Can you work these out from the model? Positions are in its coordinate system, mm. Face numbers are marked on the shaded views. A direction names the side the tool comes from. Round coordinates to 2 decimals unless told otherwise and drop trailing zeros. Order: outer loops, then holes, each group sorted by start corner. A loop starts at its lowest first (then second) coordinate and runs counter-clockwise, first axis right, second up. Notation, with made-up numbers: M 75.25,-31 L 111.25,-31 A17 cw 111.25,-16 Z; hole C 82.25,25.5 d11. An arc over 180 degrees is marked long. One line per question, with ' | ' between items.
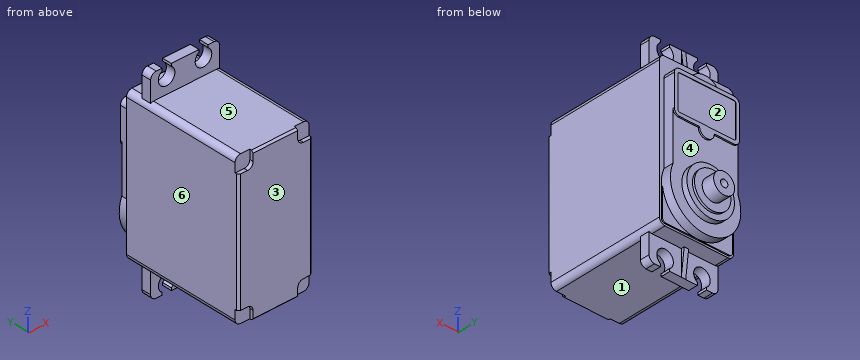
```python
from build123d import *

# Parameters (mm, degrees)
BOSS_EXTRUDE1_DEPTH  = 33.2
BOSS_EXTRUDE2_DEPTH  = 2.55
BOSS_EXTRUDE11_DEPTH = 0.3
BOSS_EXTRUDE3_DEPTH  = 2.7
SKETCH6_R            = 4.4225
BOSS_EXTRUDE4_DEPTH  = 2.5
SKETCH7_R            = 6.45
BOSS_EXTRUDE5_DEPTH  = 1.5
SKETCH8_R            = 4.95
BOSS_EXTRUDE6_DEPTH  = 0.6
SKETCH10_R           = 2.85
BOSS_EXTRUDE7_DEPTH  = 3.4
SKETCH12_R           = 1
CUT_EXTRUDE1_DEPTH   = 5
BOSS_EXTRUDE9_DEPTH  = 0.4
BOSS_EXTRUDE10_DEPTH = 0.3
CHAMFER1_SIZE        = 0.5
CUT_EXTRUDE2_DEPTH   = 1
MIRROR2_COPY_1_DEPTH = 1
BOSS_EXTRUDE12_DEPTH = 0.6


with BuildPart() as part:
    # Sketch1 → Boss-Extrude1 (new body)
    with BuildSketch(Plane(origin=(0, 0, 0), x_dir=(1, 0, 0), z_dir=(0, 1, 0))):
        with BuildLine():
            Line((-8.55, -25.58), (8.55, -25.58))
            ThreePointArc((8.55, -25.58), (9.610660172, -25.140660172), (10.05, -24.08))
            Line((10.05, -24.08), (10.05, 13.72))
            ThreePointArc((10.05, 13.72), (9.610660172, 14.780660172), (8.55, 15.22))
            Line((8.55, 15.22), (-8.55, 15.22))
            ThreePointArc((-8.55, 15.22), (-9.610660172, 14.780660172), (-10.05, 13.72))
            Line((-10.05, 13.72), (-10.05, -24.08))
            ThreePointArc((-10.05, -24.08), (-9.610660172, -25.140660172), (-8.55, -25.58))
        make_face()
    extrude(amount=BOSS_EXTRUDE1_DEPTH)

    # Sketch4 → Boss-Extrude2 (add)
    with BuildSketch(Plane(origin=(0, 26.8, 0), x_dir=(1, 0, 0), z_dir=(0, 1, 0))):
        with BuildLine():
            Line((-6.25, 22.12), (-6.25, 21.440828693))
            ThreePointArc((-6.25, 21.440828693), (-5, 17.32), (-3.75, 21.440828693))
            Line((-3.75, 21.440828693), (-3.75, 22.12))
            Line((-3.75, 22.12), (3.75, 22.12))
            Line((3.75, 22.12), (3.75, 21.440828693))
            ThreePointArc((3.75, 21.440828693), (5, 17.32), (6.25, 21.440828693))
            Line((6.25, 21.440828693), (6.25, 22.12))
            Line((6.25, 22.12), (7.85, 22.12))
            ThreePointArc((7.85, 22.12), (8.910660172, 21.680660172), (9.35, 20.62))
            Line((9.35, 20.62), (9.35, -30.98))
            ThreePointArc((9.35, -30.98), (8.910660172, -32.040660172), (7.85, -32.48))
            Line((7.85, -32.48), (6.25, -32.48))
            Line((6.25, -32.48), (6.25, -31.800828693))
            ThreePointArc((6.25, -31.800828693), (5, -27.68), (3.75, -31.800828693))
            Line((3.75, -31.800828693), (3.75, -32.48))
            Line((3.75, -32.48), (-3.75, -32.48))
            Line((-3.75, -32.48), (-3.75, -31.800828693))
            ThreePointArc((-3.75, -31.800828693), (-5, -27.68), (-6.25, -31.800828693))
            Line((-6.25, -31.800828693), (-6.25, -32.48))
            Line((-6.25, -32.48), (-7.85, -32.48))
            ThreePointArc((-7.85, -32.48), (-8.910660172, -32.040660172), (-9.35, -30.98))
            Line((-9.35, -30.98), (-9.35, 20.62))
            ThreePointArc((-9.35, 20.62), (-8.910660172, 21.680660172), (-7.85, 22.12))
            Line((-7.85, 22.12), (-6.25, 22.12))
        make_face()
    extrude(amount=BOSS_EXTRUDE2_DEPTH)

    # Sketch16 → Boss-Extrude11 (add)
    with BuildSketch(Plane(origin=(0, 33.2, 0), x_dir=(1, 0, 0), z_dir=(0, 1, 0))):
        with BuildLine():
            Line((-9.55, 13.72), (-9.55, 6.17))
            Line((-9.55, 6.17), (9.55, 6.17))
            Line((9.55, 6.17), (9.55, 13.72))
            ThreePointArc((9.55, 13.72), (9.257106781, 14.427106781), (8.55, 14.72))
            Line((8.55, 14.72), (-8.55, 14.72))
            ThreePointArc((-8.55, 14.72), (-9.257106781, 14.427106781), (-9.55, 13.72))
        make_face()
    extrude(amount=BOSS_EXTRUDE11_DEPTH)

    # Sketch5 → Boss-Extrude3 (add)
    with BuildSketch(Plane(origin=(0, 33.2, 0), x_dir=(1, 0, 0), z_dir=(0, 1, 0))):
        with BuildLine():
            Line((-8.85, 1.581128311), (-8.85, -20.08))
            ThreePointArc((-8.85, -20.08), (-8.410660172, -21.140660172), (-7.35, -21.58))
            Line((-7.35, -21.58), (7.35, -21.58))
            ThreePointArc((7.35, -21.58), (8.410660172, -21.140660172), (8.85, -20.08))
            Line((8.85, -20.08), (8.85, 1.581128311))
            ThreePointArc((8.85, 1.581128311), (0, 14.72), (-8.85, 1.581128311))
        make_face()
    extrude(amount=BOSS_EXTRUDE3_DEPTH)

    # Sketch6 → Boss-Extrude4 (add)
    with BuildSketch(Plane(origin=(0, 33.2, 0), x_dir=(1, 0, 0), z_dir=(0, 1, 0))):
        with Locations((0, -19.1575)):
            Circle(SKETCH6_R)
    extrude(amount=BOSS_EXTRUDE4_DEPTH)

    # Sketch7 → Boss-Extrude5 (add)
    with BuildSketch(Plane(origin=(0, 35.9, 0), x_dir=(1, 0, 0), z_dir=(0, 1, 0))):
        with Locations((0, 5.17)):
            Circle(SKETCH7_R)
    extrude(amount=BOSS_EXTRUDE5_DEPTH)

    # Sketch8 → Boss-Extrude6 (add)
    with BuildSketch(Plane(origin=(0, 37.4, 0), x_dir=(1, 0, 0), z_dir=(0, 1, 0))):
        with Locations((0, 5.17)):
            Circle(SKETCH8_R)
    extrude(amount=BOSS_EXTRUDE6_DEPTH)

    # Sketch10 → Boss-Extrude7 (add)
    with BuildSketch(Plane(origin=(0, 38, 0), x_dir=(1, 0, 0), z_dir=(0, 1, 0))):
        with Locations((0, 5.17)):
            Circle(SKETCH10_R)
    extrude(amount=BOSS_EXTRUDE7_DEPTH)

    # Sketch12 → Cut-Extrude1 (cut)
    with BuildSketch(Plane(origin=(0, 41.4, 0), x_dir=(1, 0, 0), z_dir=(0, 1, 0))):
        with Locations((0, 5.17)):
            Circle(SKETCH12_R)
    extrude(amount=-CUT_EXTRUDE1_DEPTH, mode=Mode.SUBTRACT)

    # Sketch13 → Boss-Extrude9 (add)
    with BuildSketch(Plane(origin=(0, 35.9, 0), x_dir=(1, 0, 0), z_dir=(0, 1, 0))):
        with BuildLine():
            Line((-8.85, -11.58), (-8.85, -20.08))
            ThreePointArc((-8.85, -20.08), (-8.410660172, -21.140660172), (-7.35, -21.58))
            Line((-7.35, -21.58), (7.35, -21.58))
            ThreePointArc((7.35, -21.58), (8.410660172, -21.140660172), (8.85, -20.08))
            Line((8.85, -20.08), (8.85, -11.58))
            ThreePointArc((8.85, -11.58), (8.410660172, -10.519339828), (7.35, -10.08))
            Line((7.35, -10.08), (2, -10.08))
            ThreePointArc((2, -10.08), (0, -8.08), (-2, -10.08))
            Line((-2, -10.08), (-7.35, -10.08))
            ThreePointArc((-7.35, -10.08), (-8.410660172, -10.519339828), (-8.85, -11.58))
        make_face()
        with BuildLine():
            Line((-7.85, -11.58), (-7.85, -20.08))
            ThreePointArc((-7.85, -20.08), (-7.703553391, -20.433553391), (-7.35, -20.58))
            Line((-7.35, -20.58), (7.35, -20.58))
            ThreePointArc((7.35, -20.58), (7.703553391, -20.433553391), (7.85, -20.08))
            Line((7.85, -20.08), (7.85, -11.58))
            ThreePointArc((7.85, -11.58), (7.703553391, -11.226446609), (7.35, -11.08))
            Line((7.35, -11.08), (-7.35, -11.08))
            ThreePointArc((-7.35, -11.08), (-7.703553391, -11.226446609), (-7.85, -11.58))
        make_face(mode=Mode.SUBTRACT)
    extrude(amount=BOSS_EXTRUDE9_DEPTH)

    # Sketch14 → Boss-Extrude10 (add)
    with BuildSketch(Plane(origin=(0, 35.9, 0), x_dir=(1, 0, 0), z_dir=(0, 1, 0))):
        with BuildLine():
            Line((-7.85, -11.58), (-7.85, -20.08))
            ThreePointArc((-7.85, -20.08), (-7.703553391, -20.433553391), (-7.35, -20.58))
            Line((-7.35, -20.58), (7.35, -20.58))
            ThreePointArc((7.35, -20.58), (7.703553391, -20.433553391), (7.85, -20.08))
            Line((7.85, -20.08), (7.85, -11.58))
            ThreePointArc((7.85, -11.58), (7.703553391, -11.226446609), (7.35, -11.08))
            Line((7.35, -11.08), (-7.35, -11.08))
            ThreePointArc((-7.35, -11.08), (-7.703553391, -11.226446609), (-7.85, -11.58))
        make_face()
    extrude(amount=BOSS_EXTRUDE10_DEPTH)

    # Chamfer1
    chamfer1_edges = [part.edges().sort_by_distance(p)[0] for p in [
        (-10.05, 0, 5.18),
        (-9.610660172, 0, -14.780660172),
        (0, 0, -15.22),
        (9.610660172, 0, -14.780660172),
        (10.05, 0, 5.18),
        (9.610660172, 0, 25.140660172),
        (0, 0, 25.58),
        (-9.610660172, 0, 25.140660172),
    ]]
    chamfer(chamfer1_edges, length=CHAMFER1_SIZE)

    # Sketch17 → Cut-Extrude2 (cut)
    with BuildSketch(Plane.XZ):
        with BuildLine():
            Line((-10.05, 21.58), (-10.05, 24.08))
            ThreePointArc((-10.05, 24.08), (-9.610660172, 25.140660172), (-8.55, 25.58))
            Line((-8.55, 25.58), (-6.05, 25.58))
            Line((-6.05, 25.58), (-6.05, 23.08))
            ThreePointArc((-6.05, 23.08), (-6.489339828, 22.019339828), (-7.55, 21.58))
            Line((-7.55, 21.58), (-10.05, 21.58))
        make_face()
    cut_extrude2 = extrude(amount=-CUT_EXTRUDE2_DEPTH, mode=Mode.SUBTRACT)

    # Mirror1: Cut-Extrude2 across plane
    add(cut_extrude2.mirror(Plane(origin=(0, 0, 0), x_dir=(0, 0, 1), z_dir=(1, 0, 0))), mode=Mode.SUBTRACT)

    # Mirror2: Cut-Extrude2 across plane
    add(cut_extrude2.mirror(Plane.XY.offset(5.18)), mode=Mode.SUBTRACT)

    # Mirror2 copy 1 sketch → Mirror2 copy 1 (cut)
    with BuildSketch(Plane(origin=(0, 0, 10.36), x_dir=(-1, 0, 0), z_dir=(0, -1, 0))):
        with BuildLine():
            Line((-10.05, 21.58), (-10.05, 24.08))
            ThreePointArc((-10.05, 24.08), (-9.610660172, 25.140660172), (-8.55, 25.58))
            Line((-8.55, 25.58), (-6.05, 25.58))
            Line((-6.05, 25.58), (-6.05, 23.08))
            ThreePointArc((-6.05, 23.08), (-6.489339828, 22.019339828), (-7.55, 21.58))
            Line((-7.55, 21.58), (-10.05, 21.58))
        make_face()
    extrude(amount=-MIRROR2_COPY_1_DEPTH, mode=Mode.SUBTRACT)

    # Sketch19 → Boss-Extrude12 (add, symmetric)
    with BuildSketch(Plane(origin=(0, 0, 0), x_dir=(0, 0, -1), z_dir=(1, 0, 0))):
        Polygon((-25.58, 30.2), (-25.58, 29.35), (-32.48, 29.35), align=None)
        Polygon((15.22, 30.2), (15.22, 29.35), (22.12, 29.35), align=None)
    extrude(amount=BOSS_EXTRUDE12_DEPTH, both=True)


solid = part.part
```
(1) Will these pins go through, and if not, where does the flat tip stop? pin 1 Ø0.6 at (x, z) = (0, -5) entering from +Y; pin 2 Ø6 at (x, y) = (7, 11) entering from -Z; pin 3 Ø5 at (x, y) = (4.5, 33.5) entering from +Z.
Final values:
pin 1: y = 36.4 | pin 2: z = -15.22 | pin 3: z = 25.58
(2) If we section it at C-C on z = -19.57: Please give me the cut outline in (x, y).
Final values:
outline: M -9.35,26.8 L -7.25,26.8 L -7.25,29.35 L -9.35,29.35 Z; M -2.75,26.8 L 2.75,26.8 L 2.75,29.35 L 0.6,29.35 L 0.6,29.66 L -0.6,29.66 L -0.6,29.35 L -2.75,29.35 Z; M 7.25,26.8 L 9.35,26.8 L 9.35,29.35 L 7.25,29.35 Z
(3) If we section it at A-A on z = 5: Please give me the cut outline in (x, y), plus the area to 3 significant figures.
Final values:
outline: M -10.05,0.5 L -9.55,0 L 9.55,0 L 10.05,0.5 L 10.05,33.2 L 8.85,33.2 L 8.85,35.9 L -8.85,35.9 L -8.85,33.2 L -10.05,33.2 Z | area: 715 mm^2
(4) If we section it at B-B on y = 13: Please give me the cut outline in (x, z).
Final values:
outline: M -10.05,-13.72 A1.5 ccw -8.55,-15.22 L 8.55,-15.22 A1.5 ccw 10.05,-13.72 L 10.05,24.08 A1.5 ccw 8.55,25.58 L -8.55,25.58 A1.5 ccw -10.05,24.08 Z
(5) Thinking about a two-plate mould opening in Z: for the marked faces 1, 2 and 3, which applies, released by +Z, released by -Z, zero draft, split by the parting line, or undercut?
Final values:
face 1: released by -Z | face 2: undercut | face 3: zero draft
(6) Please list where these lines run through material, in increasing order: probe 1 along X at (y, z) = (27.8, 29.93); probe 2 along X at (y, z) = (39.6, -5.17); probe 3 along Y at (x, z) = (-4.5, 3). Write a range as [from, to].
Final values:
probe 1: [-9.35, -7.25], [-2.75, 2.75], [7.25, 9.35] | probe 2: [-2.85, -1], [1, 2.85] | probe 3: [0, 35.9]
(7) On a 3-axis mill with a long thin cutter (end or side, diameter ignored), from which of +Z, -Z, +X, -X, +Y, -Y can I reach the whole of each face in a straight line? I mean the marked faces 4, 5 and 6. Say none if no direction works.
Final values:
face 4: +Y | face 5: +Z, +X, -X, -Y | face 6: +Z, -Z, -X, +Y, -Y
